Autodesk Inventor part; units mm, degrees
ref_plane "YZ Plane" through (0, 0, 0) normal (1, 0, 0) x (0, 1, 0)
ref_plane "XZ Plane" through (0, 0, 0) normal (0, 1, 0) x (-1, 0, 0)
ref_plane "XY Plane" through (0, 0, 0) normal (0, 0, 1) x (1, 0, 0)
sketch "Sketch1" plane through (0, 0, 0) normal (0, 1, 0) x (-1, 0, 0)
  circle A0 centre (0, 0) radius 4
  line L0 (0, -7.5056) -> (-6.5, -3.7528)
  line L1 (-6.5, -3.7528) -> (-6.5, 3.7528)
  line L2 (-6.5, 3.7528) -> (0, 7.5056)
  line L3 (0, 7.5056) -> (6.5, 3.7528)
  line L4 (6.5, 3.7528) -> (6.5, -3.7528)
  line L5 (6.5, -3.7528) -> (0, -7.5056)
  dimension "d0" = 8
  dimension "d1" = 13
extrude "Extrusion1" add sketch "Sketch1" along normal blind 5.5
sketch "Sketch2" plane through (0, 5.5, 0) normal (0, 1, 0) x (1, 0, 0)
  circle A0 centre (0, 0) radius 4
  circle A1 centre (0, 0) radius 6
  dimension "d6" = 2
extrude "Extrusion2" add sketch "Sketch2" along normal blind 1.5
fillet "Fillet1" radius 1.5 2 edges at (-6, 7, 0) (-6, 5.5, 0)
thread "Thread2"
properties part number "Mutter"
For this review, take the finished solid that the model builds, in its own axes (mm). Coordinates: 2 decimals unless noted, no trailing zeros. Loops run counter-clockwise (first coordinate to the right, second up) from the corner with the lowest first, then second, coordinate; pieces in that order, holes last. Notation, with made-up numbers: (35, -18.75) -> (88, -18.75) arc R12 ccw to (88, 0.25) -> close; hole circle Ø4 at (44.25, 88). An arc over 180 degrees is marked (long way). Write each question's results on one line, items separated by ' | '.
Q1. Add section A-A, the plane y = 2.25. State the section outline as (x, z) points, then the cut area to 3 significant figures.
Taken from the geometry:
outline: (-6.5, -3.75) -> (0, -7.51) -> (6.5, -3.75) -> (6.5, 3.75) -> (0, 7.51) -> (-6.5, 3.75) -> close; hole circle Ø8 at (0, 0) | area: 96.1 mm²
Q2. Add section B-B, the plane y = 6.5. State the section outline as (x, z) points, then the cut area to 3 significant figures.
Taken from the geometry:
outline: circle Ø11.24 at (0, 0); hole circle Ø8 at (0, 0) | area: 48.9 mm²
Q3. To check wall thickness, follow line 1 along X through (y, z) = (4, 0); line 2 along X through (y, z) = (4, -1.5); line 3 along Z through (x, y) = (-2, 4.5). State the ranges of each line that lie inside material, in increasing order. Write a range as [from, to].
Taken from the geometry:
line 1: [-6.5, -4], [4, 6.5] | line 2: [-6.5, -3.71], [3.71, 6.5] | line 3: [-6.35, -3.46], [3.46, 6.35]
Q4. For pin 1 Ø4 at (x, y) = (3.5, 2) entering from +Z; pin 2 Ø0.6 at (x, z) = (6, -4) entering from +Y; pin 3 Ø3 at (x, z) = (-5, 4.5) entering from +Y, all flat-tipped, find the tip position at first contact; note any pin that passes through.
Taken from the geometry:
pin 1: z = 6.64 | pin 2: y = 5.51 | pin 3: y = 6.81
